Geometry: final body of the model. Coordinates: model frame, mm. Face numbers are marked on the shaded views. A direction names the side the tool comes from. Round coordinates to 2 decimals unless told otherwise and drop trailing zeros. Loops run counter-clockwise (first coordinate to the right, second up) from the corner with the lowest first, then second, coordinate; pieces in that order, holes last. Notation, with made-up numbers: (38.25, 53.5) - (70.25, 53.5) arc R14 ccw to (70.25, 57.5) - close; hole circle Ø2 at (58, 30.5). An arc over 180 degrees is marked (long way). Answer in a Markdown table with one row per item. Add a question column.
from build123d import *

# Parameters (mm, degrees)
SKETCH1_R                = 2.5
BOSS_EXTRUDE1_DEPTH      = 23.375
SKETCH2_W                = 12
SKETCH2_H                = 6
BOSS_EXTRUDE2_DEPTH      = 2
SKETCH3_W                = 3
SKETCH3_H                = 6
BOSS_EXTRUDE3_DEPTH      = 6
SKETCH4_R                = 1.75
CUT_EXTRUDE1_DEPTH       = 34.725222386
FILLET1_R                = 3
CHAMFER2_SIZE            = 0.5
FILLET1_OF_MIRROR1_R     = 3
CHAMFER2_OF_MIRROR1_SIZE = 0.5


with BuildPart() as part:
    # Sketch1 → Boss-Extrude1 (new, symmetric)
    with BuildSketch(Plane(origin=(0, 0, 0), x_dir=(1, 0, 0), z_dir=(0, 1, 0))):
        with Locations(Location((0, 0, 0), (0, 0, 270))):
            Circle(SKETCH1_R)
    extrude(amount=BOSS_EXTRUDE1_DEPTH, both=True)

    # Sketch2 → Boss-Extrude2 (add)
    with BuildSketch(Plane(origin=(0, 23.375, 0), x_dir=(1, 0, 0), z_dir=(0, 1, 0))):
        Rectangle(SKETCH2_W, SKETCH2_H)
    boss_extrude2 = extrude(amount=BOSS_EXTRUDE2_DEPTH)

    # Sketch3 → Boss-Extrude3 (add)
    with BuildSketch(Plane(origin=(0, 25.375, 0), x_dir=(1, 0, 0), z_dir=(0, 1, 0))):
        with Locations((-4.5, 0)):
            Rectangle(SKETCH3_W, SKETCH3_H)
        with Locations((4.5, 0)):
            Rectangle(SKETCH3_W, SKETCH3_H)
    boss_extrude3 = extrude(amount=BOSS_EXTRUDE3_DEPTH)

    # Sketch4 → Cut-Extrude1 (cut, through all)
    with BuildSketch(Plane.ZY.offset(6)):
        with Locations((0, 28.875)):
            Circle(SKETCH4_R)
    cut_extrude1 = extrude(amount=-CUT_EXTRUDE1_DEPTH, mode=Mode.SUBTRACT)

    # Fillet1
    fillet1_edges = [part.edges().sort_by_distance(p)[0] for p in [
        (4.5, 31.375, 3),
        (4.5, 31.375, -3),
        (-4.5, 31.375, 3),
        (-4.5, 31.375, -3),
    ]]
    fillet(fillet1_edges, radius=FILLET1_R - 0.0001)  # a hair under: the kernel refuses the full size

    # Chamfer2
    chamfer2_edges = [part.edges().sort_by_distance(p)[0] for p in [
        (0, 23.375, -3),
        (0, 23.375, 3),
    ]]
    chamfer(chamfer2_edges, length=CHAMFER2_SIZE - 0.0001)  # a hair under: the kernel refuses the full size

    # Mirror1: Boss-Extrude2, Boss-Extrude3, Cut-Extrude1 across plane
    add(boss_extrude2.mirror(Plane.ZX))
    add(boss_extrude3.mirror(Plane.ZX))
    add(cut_extrude1.mirror(Plane.ZX), mode=Mode.SUBTRACT)

    # Fillet1 of Mirror1
    fillet1_of_mirror1_edges = [part.edges().sort_by_distance(p)[0] for p in [
        (4.5, -31.375, 3),
        (4.5, -31.375, -3),
        (-4.5, -31.375, 3),
        (-4.5, -31.375, -3),
    ]]
    fillet(fillet1_of_mirror1_edges, radius=FILLET1_OF_MIRROR1_R - 0.0001)  # a hair under: the kernel refuses the full size

    # Chamfer2 of Mirror1
    chamfer2_of_mirror1_edges = [part.edges().sort_by_distance(p)[0] for p in [
        (0, -23.375, -3),
        (0, -23.375, 3),
    ]]
    chamfer(chamfer2_of_mirror1_edges, length=CHAMFER2_OF_MIRROR1_SIZE - 0.0001)  # a hair under: the kernel refuses the full size


solid = part.part
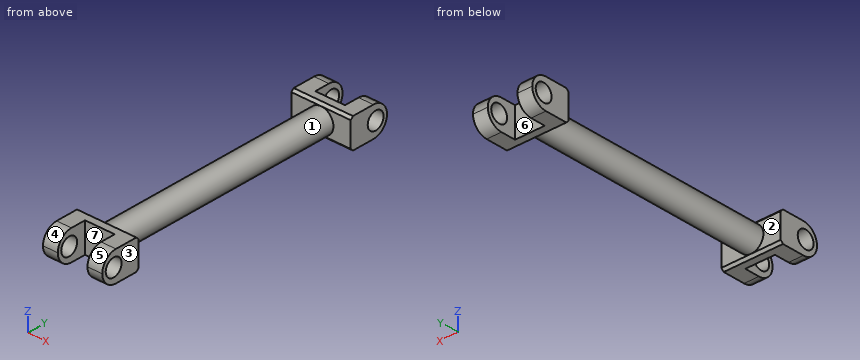
1) Contact query for flat-ended pins moving along their axis: pin 1 Ø1.8 at (x, z) = (-1.5, -0.5) entering from +Y (3 decimals); pin 2 Ø2 at (y, z) = (-28.875, 0) entering from +X; pin 3 Ø1.8 at (x, z) = (0, -1) entering from -Y (3 decimals); pin 4 Ø3 at (y, z) = (0.5, -0.5) entering from +X. Output: stop coordinate, or through.
2) Pull-direction query (Y, two-part tool) for the marked faces 1, 2, 3 and 4; classes: pulls with the +Y half, pulls with the -Y half, needs draft (parallel to the pull), parting line crosses it, or undercut.
3) Material intervals for line 1 along Y through (x, z) = (4.1, 0) (3 decimals); line 2 along Y through (x, z) = (4, -1.25) (3 decimals); line 3 along X through (y, z) = (-27, 0.75), sorted ascending. Write a range as from..to.
4) Section A-A, the plane x = 5.25. Give the number of separate pieces and of enclosed holes in the cut face, and give its area (3 significant figures).
5) Reachability of the marked faces 5, 6 and 7 from +Z, -Z, +X, -X, +Y, -Y: full face, straight path, thin tool, end or side. Return the list, or none.
6) Section C-C, the plane y = 5. Return the cut outline in (x, z).
Evaluation:
| question | item | result |
|---|---|---|
| 1 | pin 1 | stops at y = 25.375 |
| 1 | pin 2 | passes through |
| 1 | pin 3 | stops at y = -25.375 |
| 1 | pin 4 | stops at x = 2.5 |
| 2 | face 1 | undercut |
| 2 | face 2 | undercut |
| 2 | face 3 | needs draft |
| 2 | face 4 | pulls with the -Y half |
| 3 | line 1 | y = -31.375..-30.625, -27.125..-23.375, 23.375..27.125, 30.625..31.375 |
| 3 | line 2 | y = -31.102..-30.1, -27.65..-23.375, 23.375..27.65, 30.1..31.102 |
| 3 | line 3 | x = -6..-3, 3..6 |
| 4 | separate pieces | 2 |
| 4 | enclosed holes | 2 |
| 4 | area | 68.5 mm² |
| 5 | face 5 | +Z, +X, -X, -Y |
| 5 | face 6 | +Z, -Z, +Y |
| 5 | face 7 | +Z, -Z, -Y |
| 6 | outline | circle Ø5 at (0, 0) |
